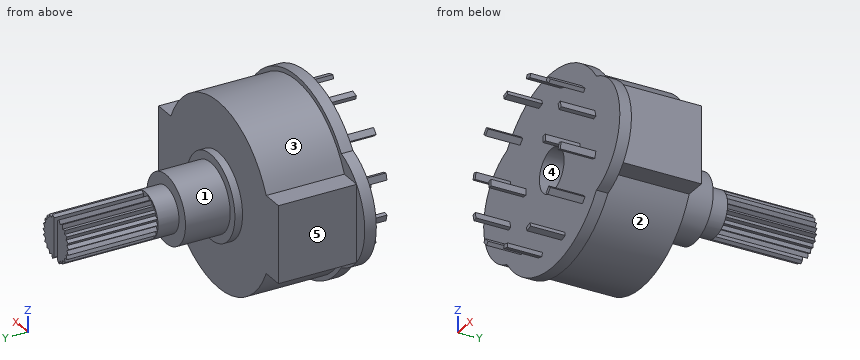
from build123d import *

# Parameters (mm, degrees)
BOSS_EXTRUDE1_DEPTH = 10.15
BOSS_EXTRUDE2_DEPTH = 1.5
SKETCH4_R           = 5.46
BOSS_EXTRUDE3_DEPTH = 1
SKETCH5_R           = 4.4
BOSS_EXTRUDE4_DEPTH = 5.8
SKETCH6_R           = 2.915
BOSS_EXTRUDE5_DEPTH = 14.32
BOSS_EXTRUDE6_DEPTH = 4.5
SKETCH8_W           = 0.5
SKETCH8_H           = 0.85
BOSS_EXTRUDE7_DEPTH = 4.5
SKETCH9_R           = 2.8
CUT_EXTRUDE1_DEPTH  = 4.5
CUT_EXTRUDE3_DEPTH  = 11.6
SKETCH10_W          = 0.8
SKETCH10_H          = 6.735502357
CUT_EXTRUDE2_DEPTH  = 11.6


with BuildPart() as part:
    # Sketch2 → Boss-Extrude1 (new body)
    with BuildSketch(Plane(origin=(0, 0, 0), x_dir=(1, 0, 0), z_dir=(0, 1, 0))):
        with BuildLine():
            Line((-13.6, 5), (-13.6, -5))
            Line((-13.6, -5), (-10.820646931, -5))
            ThreePointArc((-10.820646931, -5), (0, -11.92), (10.820646931, -5))
            Line((10.820646931, -5), (13.6, -5))
            Line((13.6, -5), (13.6, 5))
            Line((13.6, 5), (10.820646931, 5))
            ThreePointArc((10.820646931, 5), (0, 11.92), (-10.820646931, 5))
            Line((-10.820646931, 5), (-13.6, 5))
        make_face()
    extrude(amount=BOSS_EXTRUDE1_DEPTH)

    # Sketch3 → Boss-Extrude2 (add)
    with BuildSketch(Plane.XZ):
        with BuildLine():
            ThreePointArc((-10.142976429, -7.305479393), (0, -12.5), (10.142976429, -7.305479393))
            ThreePointArc((10.142976429, -7.305479393), (15.45, 0), (10.142976429, 7.305479393))
            ThreePointArc((10.142976429, 7.305479393), (0, 12.5), (-10.142976429, 7.305479393))
            ThreePointArc((-10.142976429, 7.305479393), (-15.45, 0), (-10.142976429, -7.305479393))
        make_face()
    extrude(amount=BOSS_EXTRUDE2_DEPTH)

    # Sketch4 → Boss-Extrude3 (add)
    with BuildSketch(Plane(origin=(0, 10.15, 0), x_dir=(1, 0, 0), z_dir=(0, 1, 0))):
        Circle(SKETCH4_R)
    extrude(amount=BOSS_EXTRUDE3_DEPTH)

    # Sketch5 → Boss-Extrude4 (add)
    with BuildSketch(Plane(origin=(0, 11.15, 0), x_dir=(1, 0, 0), z_dir=(0, 1, 0))):
        Circle(SKETCH5_R)
    extrude(amount=BOSS_EXTRUDE4_DEPTH)

    # Sketch6 → Boss-Extrude5 (add)
    with BuildSketch(Plane(origin=(0, 16.95, 0), x_dir=(1, 0, 0), z_dir=(0, 1, 0))):
        Circle(SKETCH6_R)
    extrude(amount=BOSS_EXTRUDE5_DEPTH)

    # Sketch7 → Boss-Extrude6 (add)
    with BuildSketch(Plane.XZ.offset(1.5)):
        Polygon((2.113087536, 9.528222971), (2.933883844, 9.307330641), (3.063820508, 9.790151999), (2.243024201, 10.011044329), align=None)
        Polygon((6.948038104, 7.548306607), (7.548422392, 6.946610084), (7.194483261, 6.593442855), (6.594098972, 7.195139378), align=None)
        Polygon((9.791330808, 3.063006225), (10.010430592, 2.241729606), (9.527326698, 2.11284738), (9.308226914, 2.934123999), align=None)
        Polygon((10.011044329, -2.243024201), (9.790151999, -3.063820508), (9.307330641, -2.933883844), (9.528222971, -2.113087536), align=None)
        Polygon((7.548306607, -6.948038104), (6.946610084, -7.548422392), (6.593442855, -7.194483261), (7.195139378, -6.594098972), align=None)
        Polygon((3.063006225, -9.791330808), (2.241729606, -10.010430592), (2.11284738, -9.527326698), (2.934123999, -9.308226914), align=None)
        Polygon((-2.243024201, -10.011044329), (-3.063820508, -9.790151999), (-2.933883844, -9.307330641), (-2.113087536, -9.528222971), align=None)
        Polygon((-6.948038104, -7.548306607), (-7.548422392, -6.946610084), (-7.194483261, -6.593442855), (-6.594098972, -7.195139378), align=None)
        Polygon((-9.791330808, -3.063006225), (-10.010430592, -2.241729606), (-9.527326698, -2.11284738), (-9.308226914, -2.934123999), align=None)
        Polygon((-10.011044329, 2.243024201), (-9.790151999, 3.063820508), (-9.307330641, 2.933883844), (-9.528222971, 2.113087536), align=None)
        Polygon((-7.548306607, 6.948038104), (-6.946610084, 7.548422392), (-6.593442855, 7.194483261), (-7.195139378, 6.594098972), align=None)
        Polygon((-3.063006225, 9.791330808), (-2.241729606, 10.010430592), (-2.11284738, 9.527326698), (-2.934123999, 9.308226914), align=None)
    extrude(amount=BOSS_EXTRUDE6_DEPTH)

    # Sketch8 → Boss-Extrude7 (add)
    with BuildSketch(Plane.XZ.offset(1.5)):
        with Locations((-6.15, 0)):
            Rectangle(SKETCH8_W, SKETCH8_H)
        with Locations((6.15, 0)):
            Rectangle(SKETCH8_W, SKETCH8_H)
    extrude(amount=BOSS_EXTRUDE7_DEPTH)

    # Sketch9 → Cut-Extrude1 (cut)
    with BuildSketch(Plane.XZ.offset(1.5)):
        Circle(SKETCH9_R)
    extrude(amount=-CUT_EXTRUDE1_DEPTH, mode=Mode.SUBTRACT)

    # Sketch11 → Cut-Extrude3 (cut)
    with BuildSketch(Plane(origin=(0, 31.27, 0), x_dir=(1, 0, 0), z_dir=(0, 1, 0))):
        with BuildLine():
            Line((-1.523472719, 1.982178316), (-1.461493827, 2.522153999))
            ThreePointArc((-1.461493827, 2.522153999), (-1.77636919, 2.311219916), (-2.061216267, 2.061216267))
            Line((-2.061216267, 2.061216267), (-1.523472719, 1.982178316))
        make_face()
        with BuildLine():
            Line((-0.958536146, 2.308940982), (-0.758913143, 2.814476122))
            ThreePointArc((-0.758913143, 2.814476122), (-1.117653146, 2.692225185), (-1.4575, 2.524464052))
            Line((-1.4575, 2.524464052), (-0.958536146, 2.308940982))
        make_face()
        with BuildLine():
            Line((-0.328276919, 2.478353136), (-0.004613782, 2.914996349))
            ThreePointArc((-0.004613782, 2.914996349), (-0.382770887, 2.889759756), (-0.754457516, 2.815673784))
            Line((-0.754457516, 2.815673784), (-0.328276919, 2.478353136))
        make_face()
        with BuildLine():
            ThreePointArc((0.75, 2.816864391), (0.378196575, 2.890361976), (0, 2.915))
            Line((0, 2.915), (0.324353838, 2.478869619))
            Line((0.324353838, 2.478869619), (0.75, 2.816864391))
        make_face()
        with BuildLine():
            ThreePointArc((1.453502522, 2.526767781), (1.113390566, 2.693990803), (0.754457516, 2.815673784))
            Line((0.754457516, 2.815673784), (0.954880417, 2.310455234))
            Line((0.954880417, 2.310455234), (1.453502522, 2.526767781))
        make_face()
        with BuildLine():
            ThreePointArc((2.057951249, 2.064476122), (1.77270883, 2.31402861), (1.4575, 2.524464052))
            Line((1.4575, 2.524464052), (1.520333473, 1.984587144))
            Line((1.520333473, 1.984587144), (2.057951249, 2.064476122))
        make_face()
        with BuildLine():
            ThreePointArc((2.522153999, 1.461493827), (2.311219916, 1.77636919), (2.061216267, 2.061216267))
            Line((2.061216267, 2.061216267), (1.982178316, 1.523472719))
            Line((1.982178316, 1.523472719), (2.522153999, 1.461493827))
        make_face()
        with BuildLine():
            ThreePointArc((2.814476122, 0.758913143), (2.692225185, 1.117653146), (2.524464052, 1.4575))
            Line((2.524464052, 1.4575), (2.308940982, 0.958536146))
            Line((2.308940982, 0.958536146), (2.814476122, 0.758913143))
        make_face()
        with BuildLine():
            ThreePointArc((2.914996349, 0.004613782), (2.889759756, 0.382770887), (2.815673784, 0.754457516))
            Line((2.815673784, 0.754457516), (2.478353136, 0.328276919))
            Line((2.478353136, 0.328276919), (2.914996349, 0.004613782))
        make_face()
        with BuildLine():
            ThreePointArc((2.816864391, -0.75), (2.890361976, -0.378196575), (2.915, 0))
            Line((2.915, 0), (2.478869619, -0.324353838))
            Line((2.478869619, -0.324353838), (2.816864391, -0.75))
        make_face()
        with BuildLine():
            ThreePointArc((2.526767781, -1.453502522), (2.693990803, -1.113390566), (2.815673784, -0.754457516))
            Line((2.815673784, -0.754457516), (2.310455234, -0.954880417))
            Line((2.310455234, -0.954880417), (2.526767781, -1.453502522))
        make_face()
        with BuildLine():
            ThreePointArc((2.064476122, -2.057951249), (2.31402861, -1.77270883), (2.524464052, -1.4575))
            Line((2.524464052, -1.4575), (1.984587144, -1.520333473))
            Line((1.984587144, -1.520333473), (2.064476122, -2.057951249))
        make_face()
        with BuildLine():
            ThreePointArc((1.461493827, -2.522153999), (1.77636919, -2.311219916), (2.061216267, -2.061216267))
            Line((2.061216267, -2.061216267), (1.523472719, -1.982178316))
            Line((1.523472719, -1.982178316), (1.461493827, -2.522153999))
        make_face()
        with BuildLine():
            ThreePointArc((0.758913143, -2.814476122), (1.117653146, -2.692225185), (1.4575, -2.524464052))
            Line((1.4575, -2.524464052), (0.958536146, -2.308940982))
            Line((0.958536146, -2.308940982), (0.758913143, -2.814476122))
        make_face()
        with BuildLine():
            ThreePointArc((0.004613782, -2.914996349), (0.382770887, -2.889759756), (0.754457516, -2.815673784))
            Line((0.754457516, -2.815673784), (0.328276919, -2.478353136))
            Line((0.328276919, -2.478353136), (0.004613782, -2.914996349))
        make_face()
        with BuildLine():
            Line((-0.324353838, -2.478869619), (-0.75, -2.816864391))
            ThreePointArc((-0.75, -2.816864391), (-0.378196575, -2.890361976), (0, -2.915))
            Line((0, -2.915), (-0.324353838, -2.478869619))
        make_face()
        with BuildLine():
            Line((-0.954880417, -2.310455234), (-1.453502522, -2.526767781))
            ThreePointArc((-1.453502522, -2.526767781), (-1.113390566, -2.693990803), (-0.754457516, -2.815673784))
            Line((-0.754457516, -2.815673784), (-0.954880417, -2.310455234))
        make_face()
        with BuildLine():
            Line((-1.520333473, -1.984587144), (-2.057951249, -2.064476122))
            ThreePointArc((-2.057951249, -2.064476122), (-1.77270883, -2.31402861), (-1.4575, -2.524464052))
            Line((-1.4575, -2.524464052), (-1.520333473, -1.984587144))
        make_face()
        with BuildLine():
            Line((-1.982178316, -1.523472719), (-2.522153999, -1.461493827))
            ThreePointArc((-2.522153999, -1.461493827), (-2.311219916, -1.77636919), (-2.061216267, -2.061216267))
            Line((-2.061216267, -2.061216267), (-1.982178316, -1.523472719))
        make_face()
        with BuildLine():
            Line((-2.308940982, -0.958536146), (-2.814476122, -0.758913143))
            ThreePointArc((-2.814476122, -0.758913143), (-2.692225185, -1.117653146), (-2.524464052, -1.4575))
            Line((-2.524464052, -1.4575), (-2.308940982, -0.958536146))
        make_face()
        with BuildLine():
            Line((-2.478353136, -0.328276919), (-2.914996349, -0.004613782))
            ThreePointArc((-2.914996349, -0.004613782), (-2.889759756, -0.382770887), (-2.815673784, -0.754457516))
            Line((-2.815673784, -0.754457516), (-2.478353136, -0.328276919))
        make_face()
        with BuildLine():
            Line((-2.478869619, 0.324353838), (-2.816864391, 0.75))
            ThreePointArc((-2.816864391, 0.75), (-2.890361976, 0.378196575), (-2.915, 0))
            Line((-2.915, 0), (-2.478869619, 0.324353838))
        make_face()
        with BuildLine():
            Line((-2.310455234, 0.954880417), (-2.526767781, 1.453502522))
            ThreePointArc((-2.526767781, 1.453502522), (-2.693990803, 1.113390566), (-2.815673784, 0.754457516))
            Line((-2.815673784, 0.754457516), (-2.310455234, 0.954880417))
        make_face()
        with BuildLine():
            Line((-1.984587144, 1.520333473), (-2.064476122, 2.057951249))
            ThreePointArc((-2.064476122, 2.057951249), (-2.31402861, 1.77270883), (-2.524464052, 1.4575))
            Line((-2.524464052, 1.4575), (-1.984587144, 1.520333473))
        make_face()
    extrude(amount=-CUT_EXTRUDE3_DEPTH, mode=Mode.SUBTRACT)

    # Sketch10 → Cut-Extrude2 (cut)
    with BuildSketch(Plane(origin=(0, 31.27, 0), x_dir=(1, 0, 0), z_dir=(0, 1, 0))):
        with Locations((0, 0.023459837)):
            Rectangle(SKETCH10_W, SKETCH10_H)
    extrude(amount=-CUT_EXTRUDE2_DEPTH, mode=Mode.SUBTRACT)


solid = part.part
Model file for the job. Use its own axes, mm. Face numbers are marked on the shaded views. A direction names the side the tool comes from. Give positions to 0.01 mm unless a question says otherwise; leave off trailing zeros. Order: outer loops, then holes, each group sorted by start corner. A loop starts at its lowest first (then second) coordinate and runs counter-clockwise, first axis right, second up. Notation, with made-up numbers: (-21.5, 29.5) - (35.5, 29.5) arc R31 ccw to (35.5, 60.5) - close; hole circle Ø1 at (48.25, 35). An arc over 180 degrees is marked (long way). Write item = value, one per line. Start each with the question number.
1. Which spindle directions (+Z, -Z, +X, -X, +Y, -Y) get a long thin tool onto all of the face, cutting with end or side? Do the marked faces 1, 2, 3, 4 and 5. Say none if no direction does.
2. Drop flat-ended pins along their axis: P1, Ø8, axis at x = 11, z = 8.5, coming from the -Y side; P2, Ø0.9, axis at y = -3.5, z = 0, coming from the +X side; P3, Ø2.5, axis at y = 23.5, z = -1, coming from the -X side (3 decimals); P4, Ø2, axis at x = -11.5, y = 8, coming from the +Z side. Give the stop position or say it passes through.
3. Cut at C-C, the plane x = -12. List the corners of the cut face in (y, z).
4. Probe line 1 along Y through (x, z) = (1.5, -10.25); line 2 along Y through (x, z) = (-1, -1); line 3 along X through (y, z) = (28.5, -1.25). List the from-to ranges inside material, lowest first.
5. Cut at A-A, the plane x = 3.5. List the corners of the cut face in (y, z).
6. Cut at B-B, the plane z = 8.25. List the corners of the cut face in (x, y).
Taken from the geometry:
q1.face_1 = +Y
q1.face_2 = -Z, +Y
q1.face_3 = +Z, +Y
q1.face_4 = -Y
q1.face_5 = +Z, -Z, -X, +Y
q2.P1 = -6
q2.P2 = 6.4
q2.P3 = -2.915
q2.P4 = 5.64
q3.outline = (-1.5, -6.41) - (0, -6.41) - (0, -5) - (10.15, -5) - (10.15, 5) - (0, 5) - (0, 6.41) - (-1.5, 6.41) - close
q4.line_1 = -1.5 to 10.15
q4.line_2 = 3 to 31.27
q4.line_3 = -2.44 to -0.4, 0.4 to 2.43
q5.outline = (-1.5, -12) - (0, -12) - (0, -11.39) - (10.15, -11.39) - (10.15, -4.19) - (11.15, -4.19) - (11.15, -2.67) - (16.95, -2.67) - (16.95, 2.67) - (11.15, 2.67) - (11.15, 4.19) - (10.15, 4.19) - (10.15, 11.39) - (0, 11.39) - (0, 12) - (-1.5, 12) - close
q6.outline = (-9.39, -1.5) - (9.39, -1.5) - (9.39, 0) - (8.6, 0) - (8.6, 10.15) - (-8.6, 10.15) - (-8.6, 0) - (-9.39, 0) - close
